```python
from build123d import *

# Parameters (mm, degrees)
F0_W     = 101.6
F0_H     = 76.2
F1_DEPTH = 38.1
F2_W     = 86.868002
F2_H     = 61.468002
F3_DEPTH = 76.201
F4_W     = 50.8
F4_H     = 25.4
F4_H_2   = 25.714025
F5_DEPTH = 76.201
F6_R     = 9.179985
F7_DEPTH = 101.601


with BuildPart() as f1:
    # F0 (on Top) → F1 (new body, symmetric)
    with BuildSketch(Plane.XY):
        Rectangle(F0_W, F0_H)
    extrude(amount=F1_DEPTH, both=True)

    # F2 (on face) → F3 (cut, through all)
    with BuildSketch(Plane.XY.offset(38.1)):
        Rectangle(F2_W, F2_H)
    extrude(amount=-F3_DEPTH, mode=Mode.SUBTRACT)

    # F4 (on face) → F5 (cut, through all)
    with BuildSketch(Plane.XZ.offset(38.1)):
        with Locations((0, 25.4)):
            Rectangle(F4_W, F4_H)
        with Locations((0, 50.957012)):
            Rectangle(F4_W, F4_H_2)
    extrude(amount=-F5_DEPTH, mode=Mode.SUBTRACT)

    # F6 (on face) → F7 (cut, through all)
    with BuildSketch(Plane.YZ.offset(50.8)):
        Circle(F6_R)
    extrude(amount=-F7_DEPTH, mode=Mode.SUBTRACT)


solid = f1.part
```
CAD build for the part. Positions are in the model's coordinates, mm. A direction names the side the tool comes from. Give positions to 0.01 mm unless a question says otherwise; leave off trailing zeros. Order: outer loops, then holes, each group sorted by start corner. A loop starts at its lowest first (then second) coordinate and runs counter-clockwise, first axis right, second up.
(1) Drill centre lines: L1, parallel to Y at x = 21, z = -13; L2, parallel to X at y = -6, z = -21; L3, parallel to Z at x = -49, y = 0. Where is each one in solid material? Low to high.
(2) Tool access for faces 4 (the flat face through (43.434, -7, 9)), 5 (the flat face through (-25.4, 34, 26)), 6 (the flat face through (50.8, 8, 9)): list every direction of +Z, -Z, +X, -X, +Y, -Y with a clear straight run to the whole face (end or side of a thin tool).
(3) Mould opens along Z. For faces 1 (the flat face through (0, -34, 12.7)), 2 (the flat face through (-25.4, -34, 26)), 3 (the cylindrical face through (47.2, -1.2, 9.1)) say: released by +Z, released by -Z, zero draft, split by the parting line, or undercut.
(4) Saw through at B-B, the plane x = 4.5. Give the cut face in (y, z), then the cut area to 3 significant figures.
(5) Saw through at D-D, the plane y = 0. Give the cut face in (x, z).
(6) Saw through at A-A, the plane y = -20. Give the cut face in (x, z), then the cut area to 3 significant figures.
(7) Flat gauge pins, fed straight in: pin 1 (16.5 mm diameter, centred on y = 0, z = 0, fed in from -X); pin 2 (3 mm diameter, centred on x = -29.5, y = 30, fed in from +Z); pin 3 (6 mm diameter, centred on x = 2.5, y = -35.5, fed in from +Z). Where does each tip first touch, or does it go through?
(8) Saw through at C-C, the plane z = 17.5. Give the cut face in (x, y).
Results found:
1. L1: y = -38.1 to -30.73, 30.73 to 38.1
1. L2: x = -50.8 to -43.43, 43.43 to 50.8
1. L3: z = -38.1 to -9.18, 9.18 to 38.1
2. face 4: +Z, -Z
2. face 5: +Z, +Y, -Y
2. face 6: +Z, -Z, +X, +Y, -Y
3. face 1: released by +Z
3. face 2: zero draft
3. face 3: undercut
4. outline: (-38.1, -38.1) - (-30.73, -38.1) - (-30.73, 12.7) - (-38.1, 12.7) - close; (30.73, -38.1) - (38.1, -38.1) - (38.1, 12.7) - (30.73, 12.7) - close
4. area: 748 mm2
5. outline: (-50.8, -38.1) - (-43.43, -38.1) - (-43.43, -9.18) - (-50.8, -9.18) - close; (-50.8, 9.18) - (-43.43, 9.18) - (-43.43, 38.1) - (-50.8, 38.1) - close; (43.43, -38.1) - (50.8, -38.1) - (50.8, -9.18) - (43.43, -9.18) - close; (43.43, 9.18) - (50.8, 9.18) - (50.8, 38.1) - (43.43, 38.1) - close
6. outline: (-50.8, -38.1) - (-43.43, -38.1) - (-43.43, 38.1) - (-50.8, 38.1) - close; (43.43, -38.1) - (50.8, -38.1) - (50.8, 38.1) - (43.43, 38.1) - close
6. area: 1,120 mm2
7. pin 1: passes through
7. pin 2: stops at z = 38.1
7. pin 3: stops at z = 12.7
8. outline: (-50.8, -38.1) - (-25.4, -38.1) - (-25.4, -30.73) - (-43.43, -30.73) - (-43.43, 30.73) - (-25.4, 30.73) - (-25.4, 38.1) - (-50.8, 38.1) - close; (25.4, -38.1) - (50.8, -38.1) - (50.8, 38.1) - (25.4, 38.1) - (25.4, 30.73) - (43.43, 30.73) - (43.43, -30.73) - (25.4, -30.73) - close
